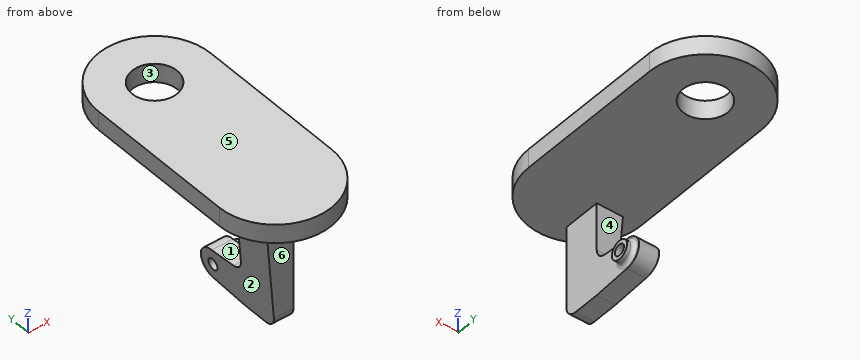
from build123d import *

# Parameters (mm, degrees)
SKETCH1_R           = 6
BOSS_EXTRUDE1_DEPTH = 5
SKETCH2_W           = 5
SKETCH2_H           = 10
BOSS_EXTRUDE2_DEPTH = 25
SKETCH3_R           = 1.5
BOSS_EXTRUDE3_DEPTH = 5
BOSS_EXTRUDE4_DEPTH = 8
BOSS_EXTRUDE5_REACH = 66.735
SKETCH5_R           = 1.5
SKETCH6_R           = 2.5
SKETCH6_R_2         = 1.5
BOSS_EXTRUDE6_DEPTH = 2
FILLET1_R           = 1
FILLET2_R           = 3


with BuildPart() as part:
    # Sketch1 → Boss-Extrude1 (new body)
    with BuildSketch(Plane.XY):
        with BuildLine():
            Line((15, 0), (15, -40))
            ThreePointArc((15, -40), (0, -55), (-15, -40))
            Line((-15, -40), (-15, 0))
            ThreePointArc((-15, 0), (0, 15), (15, 0))
        make_face()
        Circle(SKETCH1_R, mode=Mode.SUBTRACT)
    extrude(amount=BOSS_EXTRUDE1_DEPTH)

    # Sketch2 → Boss-Extrude2 (add)
    with BuildSketch(Plane(origin=(0, 0, 0), x_dir=(-1, 0, 0), z_dir=(0, 0, -1))):
        with Locations((5.75, -45)):
            Rectangle(SKETCH2_W, SKETCH2_H)
    extrude(amount=BOSS_EXTRUDE2_DEPTH)

    # Sketch3 → Boss-Extrude3 (add)
    with BuildSketch(Plane(origin=(-3.25, 0, 0), x_dir=(0, 0, -1), z_dir=(1, 0, 0))):
        with BuildLine():
            Line((24.25, -30), (25, -40))
            Line((25, -40), (15.5, -40))
            Line((15.5, -40), (16.25, -30))
            ThreePointArc((16.25, -30), (20.25, -26), (24.25, -30))
        make_face()
        with Locations(Location((20.25, -30, 0), (0, 0, 90))):
            Circle(SKETCH3_R, mode=Mode.SUBTRACT)
    extrude(amount=-BOSS_EXTRUDE3_DEPTH)

    # Sketch4 → Boss-Extrude4 (add)
    with BuildSketch(Plane.XZ.offset(50)):
        Polygon((-8.25, -25), (-8.25, 0), (-10.25, 0), align=None)
    extrude(amount=-BOSS_EXTRUDE4_DEPTH)

    # Boss-Extrude5: up to this face of the body (flat: up to its plane)
    boss_extrude5_end = Plane(part.part.faces().sort_by_distance((-9.25, -46, -12.5))[0])
    # Sketch5 → Boss-Extrude5 (add, up to the picked face)
    with BuildSketch(Plane.ZY.offset(8.25), mode=Mode.PRIVATE) as boss_extrude5_sk1:
        with BuildLine():
            Line((-24.25, -30), (-25, -40))
            Line((-25, -40), (-25, -42))
            Line((-25, -42), (0, -42))
            Line((0, -42), (0, -40))
            Line((0, -40), (-15.5, -40))
            Line((-15.5, -40), (-16.25, -30))
            ThreePointArc((-16.25, -30), (-20.25, -26), (-24.25, -30))
        make_face()
        with Locations(Location((-20.25, -30, 0), (0, 0, 90))):
            Circle(SKETCH5_R, mode=Mode.SUBTRACT)
    boss_extrude5_tool1 = split(extrude(boss_extrude5_sk1.sketch, amount=BOSS_EXTRUDE5_REACH, mode=Mode.PRIVATE), bisect_by=boss_extrude5_end, keep=Keep.BOTH, mode=Mode.PRIVATE)
    add(boss_extrude5_tool1.solids().sort_by(Axis((-8.25, -36.153945, -17.759066), (-1, 0, 0)))[0])

    # Sketch6 → Boss-Extrude6 (add)
    with BuildSketch(Plane(origin=(-3.25, 0, 0), x_dir=(0, 0, -1), z_dir=(1, 0, 0))):
        with Locations(Location((20.25, -30, 0), (0, 0, 270))):
            Circle(SKETCH6_R)
        with Locations(Location((20.25, -30, 0), (0, 0, 90))):
            Circle(SKETCH6_R_2, mode=Mode.SUBTRACT)
    extrude(amount=BOSS_EXTRUDE6_DEPTH)

    # Fillet1
    fillet1_edges = [part.edges().sort_by_distance(p)[0] for p in [
        (-3.25, -27.5, -20.25),
    ]]
    fillet(fillet1_edges, radius=FILLET1_R)

    # Fillet2
    fillet2_edges = [part.edges().sort_by_distance(p)[0] for p in [
        (-5.75, -50, -25),
        (-6.13, -40, -15.5),
    ]]
    fillet(fillet2_edges, radius=FILLET2_R)


solid = part.part
Read the model definition and answer for the solid it produces. Units are mm, in the model's axes. Face numbers are marked on the shaded views. A direction names the side the tool comes from. Round coordinates to 2 decimals unless told otherwise and drop trailing zeros. Loops run counter-clockwise (first coordinate to the right, second up) from the corner with the lowest first, then second, coordinate; pieces in that order, holes last.
Q1. Which of the six approach directions +Z, -Z, +X, -X, +Y, -Y give full straight-line access (tool end or side, diameter ignored) to the marked faces 5 and 6?
Q2. Each of these flat-tipped pins is pushed along its axis until it touches: pin 1 (5.5 mm diameter, centred on x = -8, z = -9.5, fed in from -Y); pin 2 (5 mm diameter, centred on x = -9.5, y = -24.5, fed in from -Z); pin 3 (1 mm diameter, centred on x = 2, z = -2, fed in from +Y); pin 4 (3 mm diameter, centred on y = -33, z = -21.5, fed in from +X). Where does it stop, or does it pass through?
Q3. Section A-A on x = 1 is taken. Write down the section's boundary in (y, z), and give its area (3 significant figures).
Q4. Determine the mould class of the marked faces 1, 2, 3 and 4 for opening direction Z: released by +Z, released by -Z, zero draft, split by the parting line, or undercut.
Q5. Consider probe 1 along Z at (x, y) = (-6, -30); probe 2 along Y at (x, z) = (-5.25, -20.25); probe 3 along Z at (x, y) = (7, 9.5). Determine where each line is inside the solid, lowest interval first.
Q6. Section B-B on z = -20.25 is taken. Write down the section's boundary in (x, y), and give its area (3 significant figures).
Q7. Section D-D on z = -1 is taken. Write down the section's boundary in (x, y).
Q8. Section C-C on y = -46 is taken. Write down the section's boundary in (x, z), and give its area (3 significant figures).
Output:
1. face 5: +Z, +X, -X, +Y, -Y
1. face 6: -Z, +X, -X, -Y
2. pin 1: stops at y = -50
2. pin 2: stops at z = -22.6
2. pin 3: passes through
2. pin 4: stops at x = -1.25
3. outline: (-54.97, 0) - (-5.92, 0) - (-5.92, 5) - (-54.97, 5) - close; (5.92, 0) - (14.97, 0) - (14.97, 5) - (5.92, 5) - close
3. area: 291 mm2
4. face 1: undercut
4. face 2: released by -Z
4. face 3: zero draft
4. face 4: undercut
5. probe 1: z = -24.25 to -21.75, -18.75 to -16.25, 0 to 5
5. probe 2: y = -50 to -31.5, -28.5 to -26
5. probe 3: z = 0 to 5
6. outline: (-8.63, -50) - (-3.25, -50) - (-3.25, -33.5) arc R1 cw to (-2.25, -32.5) - (-1.25, -32.5) - (-1.25, -31.5) - (-8.63, -31.5) - close; (-8.63, -28.5) - (-1.25, -28.5) - (-1.25, -27.5) - (-2.25, -27.5) arc R1 cw to (-3.25, -26.5) - (-3.25, -26) - (-8.63, -26) - close
6. area: 117 mm2
7. outline: (-10.17, -50) - (-3.25, -50) - (-3.25, -40) - (-10.17, -40) - close
8. outline: (-13.75, 0) - (-10.25, 0) - (-8.25, -25) - (-3.25, -25) - (-3.25, 0) - (13.75, 0) - (13.75, 5) - (-13.75, 5) - close
8. area: 287 mm2
